Answer from the drawing. Dimensions are ordinates in mm from the lowest x, y and z of the part. Give positions to 0.01 mm unless a question says otherwise; leave off trailing zeros. Loops run counter-clockwise (first coordinate to the right, second up) from the corner with the lowest first, then second, coordinate; pieces in that order, holes last.
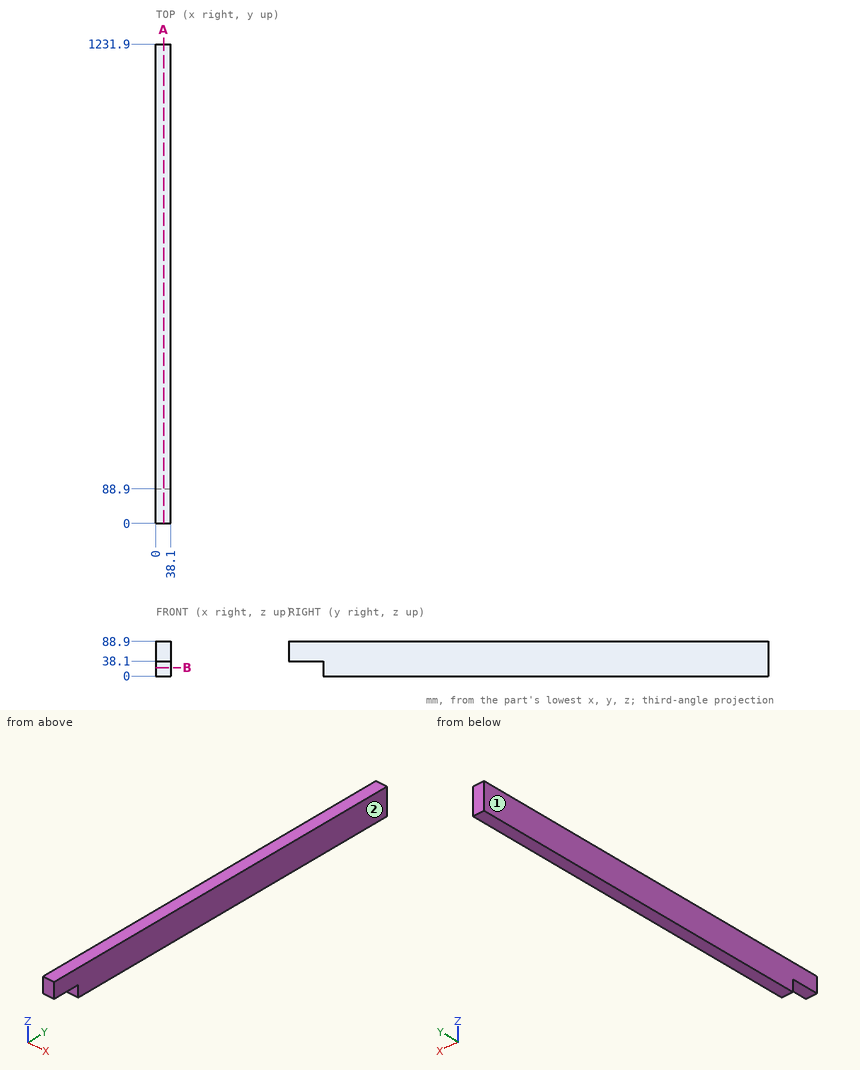
Item 1: Flat-ended cylindrical pins translate along their axes: pin 1 Ø2 at (y, z) = (1079, 32) entering from -X; pin 2 Ø11.5 at (x, z) = (21, 21) entering from -Y; pin 3 Ø19 at (x, y) = (13.5, 29) entering from -Z. Find the tip coordinate at first contact, or state that the pin passes through.
Item 2: Find section B-B, the plane z = 21.5. Write down the section's boundary in (x, y), plus the area to 3 significant figures.
Item 3: Find section A-A, the plane x = 20. Write down the section's boundary in (y, z), plus the area to 3 significant figures.
Item 4: Consider line 1 (Y direction, x = 33, z = 30). Determine where the line is inside the solid, lowest interval first.
Item 5: Determine the mould class of the marked faces 1 and 2 for opening direction X: released by +X, released by -X, zero draft, split by the parting line, or undercut.
Ans:
1. pin 1: stops at x = 0
1. pin 2: stops at y = 88.9
1. pin 3: stops at z = 38.1
2. outline: (0, 88.9) - (38.1, 88.9) - (38.1, 1231.9) - (0, 1231.9) - close
2. area: 43,500 mm2
3. outline: (0, 38.1) - (88.9, 38.1) - (88.9, 0) - (1231.9, 0) - (1231.9, 88.9) - (0, 88.9) - close
3. area: 106,000 mm2
4. line 1: y = 88.9 to 1231.9
5. face 1: released by -X
5. face 2: released by +X
